Part model, mm, in its own coordinate system. Face numbers are marked on the shaded views. A direction names the side the tool comes from. Round coordinates to 2 decimals unless told otherwise and drop trailing zeros. Order: outer loops, then holes, each group sorted by start corner. A loop starts at its lowest first (then second) coordinate and runs counter-clockwise, first axis right, second up. Notation, with made-up numbers: (47, 33.5) -> (73, 33.5) arc R11 ccw to (73, 49.5) -> close; hole circle Ø2 at (-38.5, -8.5). An arc over 180 degrees is marked (long way). Return JSON: item names as keys, results as strings. Group by question number.
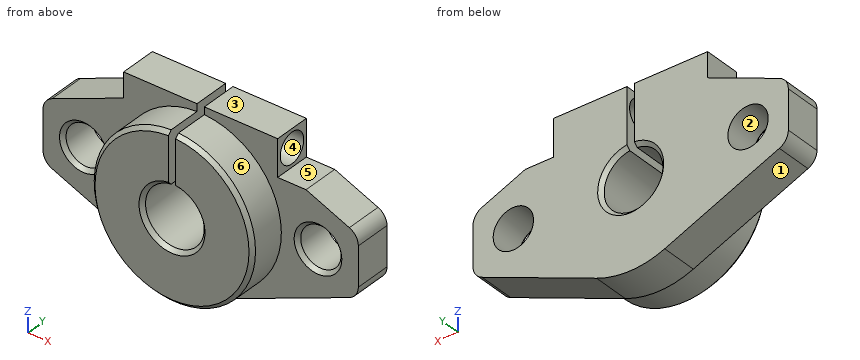
from build123d import *

# Parameters (mm, degrees)
F0_R      = 2.75
F0_R_2    = 4
F1_DEPTH  = 5
F2_R      = 11
F2_R_2    = 4
F3_DEPTH  = 5
F4_W      = 1
F4_H      = 18
F5_DEPTH  = 10.001
F6_W      = 10
F6_H      = 8.020952
F7_DEPTH  = 5
F8_W      = 5
F8_H      = 5
F9_DEPTH  = 11.001
F10_R     = 2.05
F11_DEPTH = 11
F12_SIZE  = 0.5
F13_R     = 2


with BuildPart() as f1:
    # F0 (on Front) → F1 (new body)
    with BuildSketch(Plane.XZ):
        with BuildLine():
            Line((-21.5, 4), (-21.5, -4))
            Line((-21.5, -4), (-4.638661, -11.067196))
            ThreePointArc((-4.638661, -11.067196), (0, -12), (4.638661, -11.067196))
            Line((4.638661, -11.067196), (21.5, -4))
            Line((21.5, -4), (21.5, 4))
            Line((21.5, 4), (4.638661, 11.067196))
            ThreePointArc((4.638661, 11.067196), (0, 12), (-4.638661, 11.067196))
            Line((-4.638661, 11.067196), (-21.5, 4))
        make_face()
        with Locations((-16, 0)):
            Circle(F0_R, mode=Mode.SUBTRACT)
        Circle(F0_R_2, mode=Mode.SUBTRACT)
        with Locations((16, 0)):
            Circle(F0_R, mode=Mode.SUBTRACT)
    extrude(amount=F1_DEPTH)

    # F2 (on face) → F3 (join)
    with BuildSketch(Plane.XZ.offset(5)):
        Circle(F2_R)
        Circle(F2_R_2, mode=Mode.SUBTRACT)
    extrude(amount=F3_DEPTH)

    # F4 (on face) → F5 (cut, through all)
    with BuildSketch(Plane.XZ.offset(10)):
        with Locations((0, 9)):
            Rectangle(F4_W, F4_H)
    extrude(amount=-F5_DEPTH, mode=Mode.SUBTRACT)

    # F6 (on face) → F7 (join, through all)
    with BuildSketch(Plane.XZ.offset(5)):
        with Locations((-5.5, 7.979103)):
            Rectangle(F6_W, F6_H)
        with Locations((5.5, 7.979103)):
            Rectangle(F6_W, F6_H)
    extrude(amount=-F7_DEPTH)

    # F8 (on face) → F9 (cut, through all)
    with BuildSketch(Plane.YZ.offset(10.5)):
        with Locations((-2.5, 9.489579)):
            Rectangle(F8_W, F8_H)
    extrude(amount=F9_DEPTH, mode=Mode.SUBTRACT)

    # F10 (on face) → F11 (cut, through all)
    with BuildSketch(Plane.YZ.offset(10.5)):
        with Locations((-2.5, 9.489579)):
            Circle(F10_R)
    extrude(amount=-F11_DEPTH, mode=Mode.SUBTRACT)

    # F12
    f12_edges = [f1.edges().sort_by_distance(p)[0] for p in [
        (0, 0, -4),
        (0, -10, -4),
        (0, -10, -11),
        (13.25, -5, 0),
        (-18.75, -5, 0),
    ]]
    chamfer(f12_edges, length=F12_SIZE)

    # F13
    f13_edges = [f1.edges().sort_by_distance(p)[0] for p in [
        (21.5, -2.5, -4),
        (21.5, -2.5, 4),
        (-21.5, -2.5, -4),
        (-21.5, -2.5, 4),
    ]]
    fillet(f13_edges, radius=F13_R)


solid = f1.part
(1) Pin check, flat tips, straight feed: P1, Ø2.5, axis at y = -3, z = 10.5, coming from the +X side; P2, Ø1.7, axis at y = -1.5, z = 10.5, coming from the -X side; P3, Ø4, axis at y = -4.5, z = 6, coming from the -X side. Stop position of each tip, or through.
(2) Saw through at A-A, the plane y = -3.5. List the corners of the cut face in (x, z).
(3) Probe L1, parallel to Y at x = 4, z = 9; L2, parallel to X at y = -5.5, z = 0; L3, parallel to Y at x = -10.5, z = 4.75. List the from-to ranges inside material, lowest first. Write a range as [from, to].
(4) Tool access for the marked faces 4, 5 and 6: list every direction of +Z, -Z, +X, -X, +Y, -Y with a clear straight run to the whole face (end or side of a thin tool).
(5) Saw through at B-B, the plane z = 0. State how many separate pieces and enclosed holes the cut face has, and give its area (3 significant figures).
(6) Saw through at D-D, the plane x = 0. List the corners of the cut face in (y, z).
(7) Mould opens along Z. For the marked faces 1, 2 and 3 say: pulls with the +Z half, pulls with the -Z half, needs draft (parallel to the pull), parting line crosses it, or undercut.
(8) Saw through at C-C, the plane x = -16. List the corners of the cut face in (y, z), and give its area (3 significant figures).
Results are:
{
 "1": {"P1": "stops at x = 10.5", "P2": "stops at x = -10.5", "P3": "stops at x = -20.99"},
 "2": {"outline": "(-21.5, -2.67) arc R2 ccw to (-20.27, -4.51) -> (-4.64, -11.07) arc R12 ccw to (4.64, -11.07) -> (20.27, -4.51) arc R2 ccw to (21.5, -2.67) -> (21.5, 2.67) arc R2 ccw to (20.27, 4.51) -> (14.37, 6.99) -> (10.5, 6.99) -> (10.5, 7.7) -> (0.5, 7.7) -> (0.5, 3.97) arc R4 cw (long way) to (-0.5, 3.97) -> (-0.5, 11.99) -> (-10.5, 11.99) -> (-10.5, 8.61) -> (-20.27, 4.51) arc R2 ccw to (-21.5, 2.67) -> close; (0.5, 11.28) -> (10.5, 11.28) -> (10.5, 11.99) -> (0.5, 11.99) -> close; hole circle Ø5.5 at (-16, 0); hole circle Ø5.5 at (16, 0)"},
 "3": {"L1": "y = [-10, -4.49], [-0.51, 0]", "L2": "x = [-11, -4], [4, 11]", "L3": "y = [-5, 0]"},
 "4": {"face 4": "+X", "face 5": "+Z, +X, +Y, -Y", "face 6": "-Y"},
 "5": {"separate pieces": "4", "enclosed holes": "0", "area": "189 mm^2"},
 "6": {"outline": "(-10, -10.5) -> (-9.5, -11) -> (-5, -11) -> (-5, -12) -> (0, -12) -> (0, -4.5) -> (-0.5, -4) -> (-9.5, -4) -> (-10, -4.5) -> close"},
 "7": {"face 1": "pulls with the -Z half", "face 2": "undercut", "face 3": "pulls with the +Z half"},
 "8": {"outline": "(-5, -6.31) -> (0, -6.31) -> (0, -2.75) -> (-4.5, -2.75) -> (-5, -3.25) -> close; (-5, 3.25) -> (-4.5, 2.75) -> (0, 2.75) -> (0, 6.31) -> (-5, 6.31) -> close", "area": "35.3 mm^2"}
}
